Read the model definition and answer for the solid it produces. Units are mm, in the model's axes. Face numbers are marked on the shaded views. Give positions to 0.01 mm unless a question says otherwise; leave off trailing zeros. Write each loop counter-clockwise with the first axis right and the second up, starting at its lowest first coordinate (ties: lowest second). Pieces come first, ordered by that corner, then holes. Notation, with made-up numbers: M 4,-15.75 L 36,-15.75 A26 cw 36,11.25 Z; hole C 35,84.5 d6. An arc over 180 degrees is marked long. Use a Markdown table: item, result. Add a question column.
Item 1: The mould has two halves that part along X. Classify the marked faces 1, 2, 3 and 4: pulls with the +X half, pulls with the -X half, needs draft (parallel to the pull), parting line crosses it, or undercut.
Item 2: Given P1, Ø2.5, axis at x = -2, z = -97.5, coming from the +Y side; P2, Ø3, axis at x = 98.775, z = -133.7, coming from the +Y side; P3, Ø6, axis at x = 30.5, z = 25.5, coming from the +Y side, each flat-ended and moving along its own axis, determine where each tip first touches the part or whether it passes through.
Item 3: Consider probe 1 along X at (y, z) = (94.25, -133.7) (3 decimals); probe 2 along X at (y, z) = (22.5, 31.5) (3 decimals); probe 3 along Z at (x, y) = (-94.5, 84) (3 decimals). Determine where each line is inside the solid, lowest interval first. Write a range as [from, to].
Item 4: A cutting plane is placed at A-A on y = 49.5. Determine the outline of the cut face in (x, z) (3 decimals), then the cut area to 3 significant figures.
from build123d import *

# Parameters (mm, degrees)
SKETCH2_W                                = 203.2
SKETCH2_H                                = 273.05
BOX_BASE_DEPTH                           = 6.35
SKETCH2_3_W                              = 209.55
SKETCH2_3_H                              = 279.4
SKETCH2_3_W_2                            = 203.2
SKETCH2_3_H_2                            = 273.05
BOX_WALL_HEIGHT_DEPTH                    = 98.425
SKETCH9_R                                = 2.5273
BOSS_EXTRUDE4_DEPTH                      = 12
FILLET2_R                                = 1.5875
LID_MOUNTING_HEAT_SET_INSERT_HOLES_D     = 5.0546
LID_MOUNTING_HEAT_SET_INSERT_HOLES_DEPTH = 8.89
LID_MOUNTING_HEAT_SET_INSERT_HOLES_TIP   = 1.518555042
SKETCH14_R                               = 2.5273
MME_42_MOUNTING_PEGS_DEPTH               = 10
FILLET3_R                                = 1.5875
FILLET5_R                                = 1.5875
SKETCH19_R                               = 7.7390625
CUT_EXTRUDE2_DEPTH                       = 3.175


with BuildPart() as part:
    # Sketch2 → Box Base (new body)
    with BuildSketch(Plane(origin=(0, 0, 0), x_dir=(1, 0, 0), z_dir=(0, 1, 0))):
        Rectangle(SKETCH2_W, SKETCH2_H)
    extrude(amount=BOX_BASE_DEPTH)

    # Sketch2<3> → Box Wall height (add)
    with BuildSketch(Plane(origin=(0, 0, 0), x_dir=(1, 0, 0), z_dir=(0, 1, 0))):
        Rectangle(SKETCH2_3_W, SKETCH2_3_H)
        Rectangle(SKETCH2_3_W_2, SKETCH2_3_H_2, mode=Mode.SUBTRACT)
    extrude(amount=BOX_WALL_HEIGHT_DEPTH)

    # Sketch9 → Boss-Extrude4 (add)
    with BuildSketch(Plane(origin=(0, 98.425, 0), x_dir=(1, 0, 0), z_dir=(0, 1, 0))):
        with BuildLine():
            ThreePointArc((-93.481666929, -136.525), (-94.532359313, -129.457359313), (-101.6, -128.406666929))
            Line((-101.6, -128.406666929), (-101.6, -136.525))
            Line((-101.6, -136.525), (-93.481666929, -136.525))
        make_face()
        with Locations((-98.775, -133.7)):
            Circle(SKETCH9_R, mode=Mode.SUBTRACT)
        with Locations((-98.775, -133.7)):
            Circle(SKETCH9_R)
        Polygon((-101.6, -136.525), (-101.6, -128.406666929), (-104.775, -128.406666929), (-104.775, -139.7), (-93.481666929, -139.7), (-93.481666929, -136.525), align=None)
        with BuildLine():
            ThreePointArc((101.6, -128.406666929), (94.532359313, -129.457359313), (93.481666929, -136.525))
            Line((93.481666929, -136.525), (101.6, -136.525))
            Line((101.6, -136.525), (101.6, -128.406666929))
        make_face()
        with Locations((98.775, -133.7)):
            Circle(SKETCH9_R, mode=Mode.SUBTRACT)
        with Locations((98.775, -133.7)):
            Circle(SKETCH9_R)
        Polygon((101.6, -136.525), (93.481666929, -136.525), (93.481666929, -139.7), (104.775, -139.7), (104.775, -128.406666929), (101.6, -128.406666929), align=None)
        Polygon((93.481666929, 139.7), (93.481666929, 136.525), (101.6, 136.525), (101.6, 128.406666929), (104.775, 128.406666929), (104.775, 139.7), align=None)
        with BuildLine():
            Line((101.6, 136.525), (93.481666929, 136.525))
            ThreePointArc((93.481666929, 136.525), (94.532359313, 129.457359313), (101.6, 128.406666929))
            Line((101.6, 128.406666929), (101.6, 136.525))
        make_face()
        with Locations((98.775, 133.7)):
            Circle(SKETCH9_R, mode=Mode.SUBTRACT)
        with Locations((98.775, 133.7)):
            Circle(SKETCH9_R)
        with BuildLine():
            Line((-101.6, 136.525), (-101.6, 128.406666929))
            ThreePointArc((-101.6, 128.406666929), (-94.532359313, 129.457359313), (-93.481666929, 136.525))
            Line((-93.481666929, 136.525), (-101.6, 136.525))
        make_face()
        with Locations((-98.775, 133.7)):
            Circle(SKETCH9_R, mode=Mode.SUBTRACT)
        with Locations((-98.775, 133.7)):
            Circle(SKETCH9_R)
        Polygon((-104.775, 128.406666929), (-101.6, 128.406666929), (-101.6, 136.525), (-93.481666929, 136.525), (-93.481666929, 139.7), (-104.775, 139.7), align=None)
    extrude(amount=-BOSS_EXTRUDE4_DEPTH)

    # Fillet2
    fillet2_edges = [part.edges().sort_by_distance(p)[0] for p in [
        (-93.481666929, 92.425, -136.525),
        (-101.6, 92.425, -128.406666929),
        (-93.481666929, 92.425, 136.525),
        (-101.6, 92.425, 128.406666929),
        (93.481666929, 92.425, 136.525),
        (101.6, 92.425, 128.406666929),
        (101.6, 92.425, -128.406666929),
        (93.481666929, 92.425, -136.525),
    ]]
    fillet(fillet2_edges, radius=FILLET2_R)

    # Lid Mounting heat Set Insert Holes
    with Locations(Plane(origin=(0, 98.425, 0), x_dir=(1, 0, 0), z_dir=(0, 1, 0))):
        with Locations((98.775, 133.7), (-98.775, 133.7), (-98.775, -133.7), (98.775, -133.7)):
            Hole(LID_MOUNTING_HEAT_SET_INSERT_HOLES_D / 2, depth=LID_MOUNTING_HEAT_SET_INSERT_HOLES_DEPTH)
            with Locations((0, 0, -(LID_MOUNTING_HEAT_SET_INSERT_HOLES_DEPTH + LID_MOUNTING_HEAT_SET_INSERT_HOLES_TIP / 2))):  # 118° drill point
                Cone(0, LID_MOUNTING_HEAT_SET_INSERT_HOLES_D / 2, LID_MOUNTING_HEAT_SET_INSERT_HOLES_TIP, mode=Mode.SUBTRACT)

    # Sketch14 → MME-42 Mounting Pegs (add)
    with BuildSketch(Plane(origin=(0, 6.35, 0), x_dir=(1, 0, 0), z_dir=(0, 1, 0))):
        with BuildLine():
            Line((-4.343000027, -91.236739798), (-4.343000027, -103.581260202))
            ThreePointArc((-4.343000027, -103.581260202), (5.958999973, -97.409), (-4.343000027, -91.236739798))
        make_face()
        with Locations(Location((-1.041000027, -97.409, 0), (0, 0, 270))):
            Circle(SKETCH14_R, mode=Mode.SUBTRACT)
        with BuildLine():
            ThreePointArc((23.342999973, -91.236739798), (13.040999973, -97.409), (23.342999973, -103.581260202))
            Line((23.342999973, -103.581260202), (23.342999973, -91.236739798))
        make_face()
        with Locations(Location((20.040999973, -97.409, 0), (0, 0, 270))):
            Circle(SKETCH14_R, mode=Mode.SUBTRACT)
        with BuildLine():
            Line((-4.343000027, 102.565260202), (-4.343000027, 90.220739798))
            ThreePointArc((-4.343000027, 90.220739798), (5.958999973, 96.393), (-4.343000027, 102.565260202))
        make_face()
        with Locations(Location((-1.041000027, 96.393, 0), (0, 0, 270))):
            Circle(SKETCH14_R, mode=Mode.SUBTRACT)
        with BuildLine():
            ThreePointArc((23.342999973, 102.565260202), (13.040999973, 96.393), (23.342999973, 90.220739798))
            Line((23.342999973, 90.220739798), (23.342999973, 102.565260202))
        make_face()
        with Locations(Location((20.040999973, 96.393, 0), (0, 0, 270))):
            Circle(SKETCH14_R, mode=Mode.SUBTRACT)
    extrude(amount=MME_42_MOUNTING_PEGS_DEPTH)

    # Fillet3
    fillet3_edges = [part.edges().sort_by_distance(p)[0] for p in [
        (5.958999973, 6.35, 97.409),
        (13.040999973, 6.35, 97.409),
        (5.958999973, 6.35, -96.393),
        (13.040999973, 6.35, -96.393),
    ]]
    fillet(fillet3_edges, radius=FILLET3_R)

    # Fillet5
    fillet5_edges = [part.edges().sort_by_distance(p)[0] for p in [
        (0, 6.35, 136.525),
        (101.6, 6.35, 0),
        (0, 6.35, -136.525),
        (-101.6, 6.35, 0),
    ]]
    fillet(fillet5_edges, radius=FILLET5_R)

    # Sketch19 → Cut-Extrude2 (cut)
    with BuildSketch(Plane.XY.offset(139.7)):
        with Locations((-11.963000027, 19.398)):
            Circle(SKETCH19_R)
        with Locations((9.499999973, 24.478)):
            Circle(SKETCH19_R)
        with Locations((30.962999973, 19.398)):
            Circle(SKETCH19_R)
    extrude(amount=-CUT_EXTRUDE2_DEPTH, mode=Mode.SUBTRACT)


solid = part.part
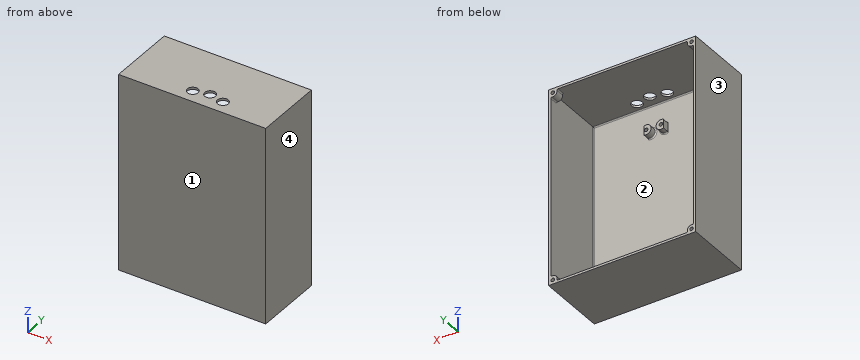
Filled in:
| question | item | result |
|---|---|---|
| 1 | face 1 | needs draft |
| 1 | face 2 | undercut |
| 1 | face 3 | pulls with the -X half |
| 1 | face 4 | pulls with the +X half |
| 2 | P1 | y = 16.35 |
| 2 | P2 | y = 88.92 |
| 2 | P3 | y = 6.35 |
| 3 | probe 1 | [-104.775, -101.302], [-96.248, -92.775], [92.775, 96.248], [101.302, 104.775] |
| 3 | probe 2 | [-104.775, -101.6], [101.6, 104.775] |
| 3 | probe 3 | [-139.7, -136.525], [136.525, 139.7] |
| 4 | outline | M -104.775,-139.7 L 104.775,-139.7 L 104.775,139.7 L -104.775,139.7 Z; hole M -101.6,-136.525 L 101.6,-136.525 L 101.6,136.525 L -101.6,136.525 Z |
| 4 | area | 3,060 mm² |
